from build123d import *

# Parameters (mm, degrees)
F0_W     = 14
F0_H     = 49.101681
F0_R     = 3.5
F0_R_2   = 3
F0_R_3   = 2.5
F0_R_4   = 2
F0_R_5   = 1.5
F0_R_6   = 1
F0_R_7   = 0.5
F1_DEPTH = 3
F2_DEPTH = 6


with BuildPart() as f1:
    # F0 (on Top) → F1 (new body)
    with BuildSketch(Plane.XY):
        with Locations((0, -8.822086)):
            Rectangle(F0_W, F0_H)
        with Locations((0, -26.690952)):
            Circle(F0_R, mode=Mode.SUBTRACT)
        with Locations((0, -17.690952)):
            Circle(F0_R_2, mode=Mode.SUBTRACT)
        with Locations((0, -9.690952)):
            Circle(F0_R_3, mode=Mode.SUBTRACT)
        with Locations((0, -2.690952)):
            Circle(F0_R_4, mode=Mode.SUBTRACT)
        with Locations((0, 3.309048)):
            Circle(F0_R_5, mode=Mode.SUBTRACT)
        with Locations((0, 8.309048)):
            Circle(F0_R_6, mode=Mode.SUBTRACT)
        with Locations((0, 12.309048)):
            Circle(F0_R_7, mode=Mode.SUBTRACT)
    extrude(amount=F1_DEPTH)

    # F0 (on Top) → F2 (join)
    with BuildSketch(Plane.XY):
        with Locations((0, -26.690952)):
            Circle(F0_R)
        with Locations((0, -17.690952)):
            Circle(F0_R_2)
        with Locations((0, -9.690952)):
            Circle(F0_R_3)
        with Locations((0, -2.690952)):
            Circle(F0_R_4)
        with Locations((0, 3.309048)):
            Circle(F0_R_5)
        with Locations((0, 8.309048)):
            Circle(F0_R_6)
        with Locations((0, 12.309048)):
            Circle(F0_R_7)
    extrude(amount=F2_DEPTH)


solid = f1.part
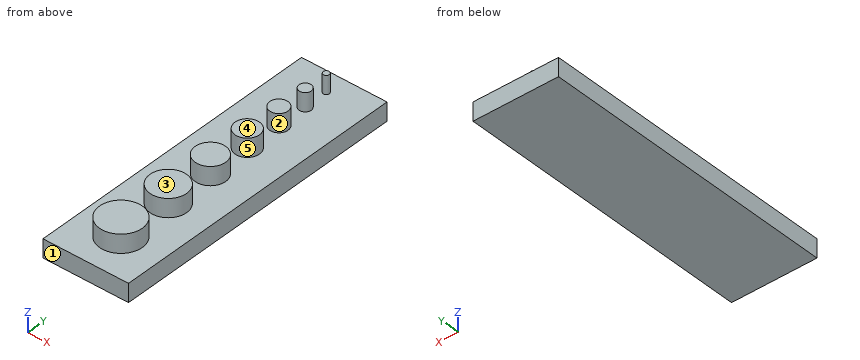
Input: part model. Units: mm. Frame: model coordinates. Face numbers are marked on the shaded views. A direction names the side the tool comes from. Round coordinates to 2 decimals unless told otherwise and drop trailing zeros. Order: outer loops, then holes, each group sorted by start corner. A loop starts at its lowest first (then second) coordinate and runs counter-clockwise, first axis right, second up.
1. Material intervals for line 1 (Z direction, x = 2, y = 1); line 2 (X direction, y = 9, z = 5.45); line 3 (X direction, y = 12, z = 4.45), sorted ascending.
The answers:
line 1: z = 0 to 3
line 2: x = -0.72 to 0.72
line 3: x = -0.39 to 0.39
2. Mould query, pull axis Y, two halves, no side actions, for the marked faces 1, 2 and 3. Classes: released by +Y, released by -Y, zero draft, split by the parting line, or undercut.
The answers:
face 1: released by -Y
face 2: undercut
face 3: zero draft
3. Pin query (flat end, axial travel): P1, Ø2, axis at y = -9, z = 5.5, coming from the -X side; P2, Ø1, axis at x = -4, y = -13.5, coming from the +Z side. Return the tip coordinate at first contact, or that it passes through.
The answers:
P1: stops at x = -2.5
P2: stops at z = 3
4. Cut plane C-C, the plane y = 10. Output: boundary loops of the cut face in (x, z), then the cut area to 3 significant figures.
The answers:
outline: (-7, 0) - (7, 0) - (7, 3) - (-7, 3) - close
area: 42.0 mm2
5. Cut plane B-B, the plane z = 3.65. Output: boundary loops of the cut face in (x, y).
The answers:
outline: circle Ø7 at (0, -26.69); circle Ø6 at (0, -17.69); circle Ø5 at (0, -9.69); circle Ø4 at (0, -2.69); circle Ø3 at (0, 3.31); circle Ø2 at (0, 8.31); circle Ø1 at (0, 12.31)
6. Cut plane D-D, the plane y = 4. Output: boundary loops of the cut face in (x, z), then the cut area to 3 significant figures.
The answers:
outline: (-7, 0) - (7, 0) - (7, 3) - (1.33, 3) - (1.33, 6) - (-1.33, 6) - (-1.33, 3) - (-7, 3) - close
area: 50.0 mm2
7. Set-up query: the marked faces 4 and 5. Return all of +Z, -Z, +X, -X, +Y, -Y with unobstructed straight access to the full face (end or side cutting, diameter ignored); none if empty.
The answers:
face 4: +Z, +X, -X, +Y, -Y
face 5: +Z
